Read the model definition and answer for the solid it produces. Units are mm, in the model's axes. Coordinates: 2 decimals unless noted, no trailing zeros. Loops run counter-clockwise (first coordinate to the right, second up) from the corner with the lowest first, then second, coordinate; pieces in that order, holes last.
Q1. Section D-D (z = 2.75) is taken. Give the vertices of the cut face in (x, y).
Q2. Section C-C (x = -3) is taken. Give the vertices of the cut face in (y, z).
Q3. Flat-ended cylindrical pins translate along their axes: P1, Ø1, axis at x = 1.5, z = -1, coming from the -Y side; P2, Ø1.8, axis at x = 0, y = 66, coming from the +Z side; P3, Ø4, axis at y = 29.5, z = -2.5, coming from the -X side. Find the tip coordinate at first contact, or state that the pin passes through.
Q4. Section A-A (z = 0) is taken. Give the vertices of the cut face in (x, y), then the cut area to 3 significant figures.
Q5. Section B-B (x = 0) is taken. Give the vertices of the cut face in (y, z).
Q6. Straight lines are drawn through the part: line 1 (Y direction, x = -3.5, z = 0); line 2 (Y direction, x = -1, z = 3.75); line 3 (Y direction, x = -0.75, z = -2.75). For each, find the intervals that lie inside material, in ascending order.
from build123d import *

# Parameters (mm, degrees)
SKETCH1_R               = 4
BOSS_EXTRUDE1_DEPTH     = 69.5
CUT_EXTRUDE1_DEPTH      = 79.218588868
CUT_EXTRUDE1_DEPTH_BACK = 79.218588868
SKETCH2_R               = 1.5
CUT_EXTRUDE2_DEPTH      = 70.729835906
CUT_EXTRUDE2_DEPTH_BACK = 70.729835906
SKETCH3_R               = 1.5
CUT_EXTRUDE3_DEPTH      = 70.729835906
CUT_EXTRUDE3_DEPTH_BACK = 70.729835906
SKETCH4_R               = 1.5


with BuildPart() as part:
    # Sketch1 → Boss-Extrude1 (new body)
    with BuildSketch(Plane(origin=(0, 0, 0), x_dir=(1, 0, 0), z_dir=(0, 1, 0))):
        with Locations(Location((0, 0, 0), (0, 0, 270))):
            Circle(SKETCH1_R)
    extrude(amount=BOSS_EXTRUDE1_DEPTH)

    # Sketch2 → Cut-Extrude1 (cut, two sides: drawn at the far end of the back side and taken through both)
    with BuildSketch(Plane(origin=(-34.800875944, 1.701477372, 0), x_dir=(1, 0, 0), z_dir=(0, 0, 1)).offset(-CUT_EXTRUDE1_DEPTH_BACK)):
        with Locations(Location((34.800875944, 2.798522628, 0), (0, 0, 90.000000025))):
            Circle(SKETCH2_R)
        with Locations(Location((34.800875944, 12.798522628, 0), (0, 0, 90.000000025))):
            Circle(SKETCH2_R)
    extrude(amount=CUT_EXTRUDE1_DEPTH + CUT_EXTRUDE1_DEPTH_BACK, mode=Mode.SUBTRACT)

    # Sketch3 → Cut-Extrude2 (cut, two sides: drawn at the far end of the back side and taken through both)
    with BuildSketch(Plane.XY.offset(-CUT_EXTRUDE2_DEPTH_BACK)):
        with Locations(Location((0, 66, 0), (0, 0, 90.000000025))):
            Circle(SKETCH3_R)
    extrude(amount=CUT_EXTRUDE2_DEPTH + CUT_EXTRUDE2_DEPTH_BACK, mode=Mode.SUBTRACT)

    # Sketch4 → Cut-Extrude3 (cut, two sides: drawn at the far end of the back side and taken through both)
    with BuildSketch(Plane(origin=(0, 0, 0), x_dir=(0, 0, -1), z_dir=(1, 0, 0)).offset(-CUT_EXTRUDE3_DEPTH_BACK)):
        with Locations((0, 62.2)):
            Circle(SKETCH4_R)
    extrude(amount=CUT_EXTRUDE3_DEPTH + CUT_EXTRUDE3_DEPTH_BACK, mode=Mode.SUBTRACT)


solid = part.part
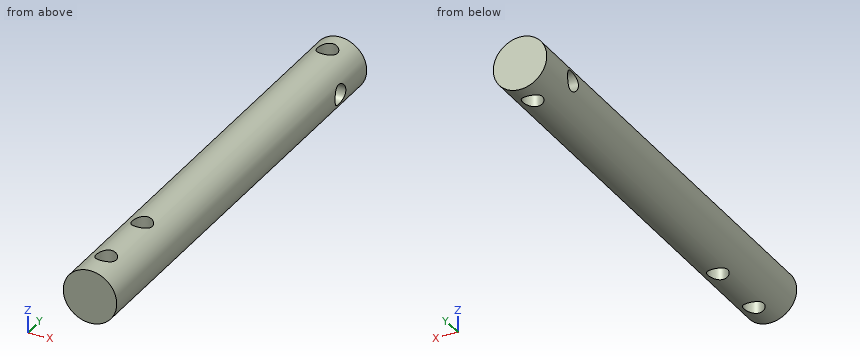
Numbers:
1. outline: (-2.9, 0) - (2.9, 0) - (2.9, 69.5) - (-2.9, 69.5) - close; hole circle Ø3 at (0, 4.5); hole circle Ø3 at (0, 14.5); hole circle Ø3 at (0, 66)
2. outline: (0, -2.65) - (69.5, -2.65) - (69.5, 2.65) - (0, 2.65) - close; hole circle Ø3 at (62.2, 0)
3. P1: stops at y = 0
3. P2: passes through
3. P3: stops at x = -3.97
4. outline: (-4, 0) - (4, 0) - (4, 60.7) - (-4, 60.7) - close; (-4, 63.7) - (4, 63.7) - (4, 69.5) - (-4, 69.5) - close; hole circle Ø3 at (0, 4.5); hole circle Ø3 at (0, 14.5); hole circle Ø3 at (0, 66)
4. area: 511 mm2
5. outline: (0, -4) - (3, -4) - (3, 4) - (0, 4) - close; (6, -4) - (13, -4) - (13, 4) - (6, 4) - close; (16, -4) - (64.5, -4) - (64.5, 4) - (16, 4) - close; (67.5, -4) - (69.5, -4) - (69.5, 4) - (67.5, 4) - close; hole circle Ø3 at (62.2, 0)
6. line 1: y = 0 to 60.7, 63.7 to 69.5
6. line 2: y = 0 to 3.38, 5.62 to 13.38, 15.62 to 64.88, 67.12 to 69.5
6. line 3: y = 0 to 3.2, 5.8 to 13.2, 15.8 to 64.7, 67.3 to 69.5
